Autodesk Inventor part; units mm, degrees
ref_plane "YZ Plane" through (0, 0, 0) normal (1, 0, 0) x (0, 1, 0)
ref_plane "XZ Plane" through (0, 0, 0) normal (0, 1, 0) x (-1, 0, 0)
ref_plane "XY Plane" through (0, 0, 0) normal (0, 0, 1) x (1, 0, 0)
sketch "Sketch2" plane through (0, 0, 0) normal (1, 0, 0) x (0, 1, 0)
  line L0 (0, 0) -> (0, -25.4)
  arc A0 (-1.9226, -30.6595) -> (0, -25.4) centre (-8.1552, -25.4) ccw
  line L1 (-1.9226, -30.6595) -> (-29.0367, -62.7904)
  arc A1 (-29.0367, -62.7904) -> (-32.8676, -73.2701) centre (-16.618, -73.2701) ccw
  line L2 (-32.8676, -73.2701) -> (-32.8676, -76.4451)
  dimension "d3" = 25.4
  dimension "d4" = 8.1552
  dimension "d5" = 16.2496
  dimension "d6" = 3.175
  dimension "d7" = 32.8676
sketch "Sketch3" plane through (0, 0, 0) normal (0, 0, 1) x (1, 0, 0)
  circle A0 centre (0, 0) radius 1
  dimension "d8" = 2
sweep "Sweep1" add profiles "Sketch3" path "Sketch2"
sketch "Sketch9" plane through (0, 0, 0) normal (1, 0, 0) x (0, 1, 0)
  line L0 (-33.8676, -76.4451) -> (-31.8676, -76.4451)
  arc A0 (-33.8676, -76.4451) -> (-31.8676, -76.4451) centre (-32.8676, -76.4451) ccw
  line L1 (-31.8676, -73.2701) -> (-31.8676, -76.4451)
  line L2 (-31.8676, -76.4451) -> (-33.8676, -76.4451)
  point P0 (0, 0)
revolve "Revolution2" add sketch "Sketch9" angle 180 mid plane about axis through (0, -33.8676, -76.4451) along (0, 1, 0)
properties part number "2mmToDive" material "Brass, Soft Yellow, Welded"
Model file for the job. Use its own axes, mm. A direction names the side the tool comes from. Round coordinates to 2 decimals unless told otherwise and drop trailing zeros. Write each loop counter-clockwise with the first axis right and the second up, starting at its lowest first coordinate (ties: lowest second). Pieces come first, ordered by that corner, then holes. Notation, with made-up numbers: M -16,2.25 L -6,2.25 A11 ccw -6,22.25 Z; hole C 71.25,-34 d7. An arc over 180 degrees is marked long. Put each result on its own line as item: value.
Item 1: Probe L1, parallel to X at y = -10, z = -40; L2, parallel to Y at x = -0.6, z = -9; L3, parallel to Z at x = 0.05, y = -9. List the from-to ranges inside material, lowest first. Write a range as from..to.
Responses:
L1: -0.99..0.99
L2: -0.8..0.8
L3: -40.6..-37.5
Item 2: Tool access for faces 1 (the flat face through (0, 0, 0)), 2 (the cylindrical face through (0, 1, -13)): list every direction of +Z, -Z, +X, -X, +Y, -Y with a clear straight run to the whole face (end or side of a thin tool).
Responses:
face 1: +Z, +X, -X, +Y, -Y
face 2: +Z
Item 3: Cut at A-A (z = -8.5). List the corners of the cut face in (x, y).
Responses:
outline: C 0,0 d2
